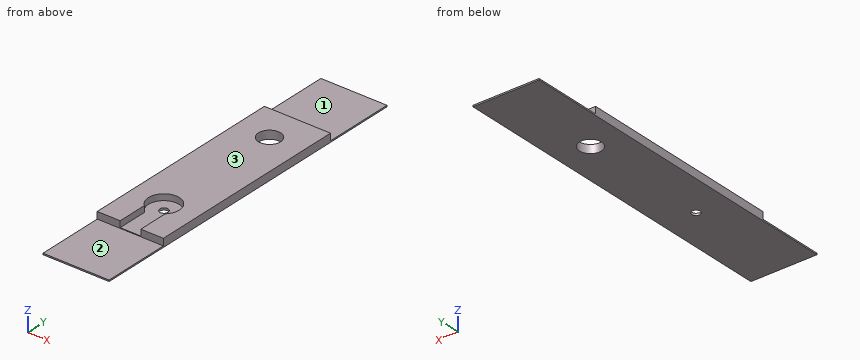
```python
from build123d import *

# Parameters (mm, degrees)
SKETCH_W        = 48
SKETCH_H        = 250.999997
SKETCH_R        = 8.05
SKETCH_R_2      = 3.05
PAD_DEPTH       = 6
POCKET_DEPTH    = 4.5
SKETCH002_W     = 48.1
SKETCH002_H     = 48.999997
POCKET001_DEPTH = 5.001
SKETCH003_W     = 48.1
SKETCH003_H     = 52
POCKET002_DEPTH = 5.001


with BuildPart() as part:
    # Sketch → Pad (new body)
    with BuildSketch(Plane.XY):
        with Locations((-24, 125.499994)):
            Rectangle(SKETCH_W, SKETCH_H)
        with Locations((-24, 174.761047)):
            Circle(SKETCH_R, mode=Mode.SUBTRACT)
        with Locations((-24, 79.409981)):
            Circle(SKETCH_R_2, mode=Mode.SUBTRACT)
    extrude(amount=-PAD_DEPTH)

    # Sketch001 → Pocket (cut)
    with BuildSketch(Plane.XY):
        with BuildLine():
            Line((-31.346662, 47.787562), (-16.346662, 47.787562))
            Line((-16.346662, 47.787562), (-16.346662, 71.017092))
            ThreePointArc((-16.346662, 71.017092), (-24.104532, 90.522743), (-31.346662, 70.819786))
            Line((-31.346662, 70.819786), (-31.346662, 47.787562))
        make_face()
    extrude(amount=-POCKET_DEPTH, mode=Mode.SUBTRACT)

    # Sketch002 → Pocket001 (cut, through all)
    with BuildSketch(Plane.XY.offset(-5)):
        with Locations((-23.95, 24.499994)):
            Rectangle(SKETCH002_W, SKETCH002_H)
    extrude(amount=POCKET001_DEPTH, mode=Mode.SUBTRACT)

    # Sketch003 → Pocket002 (cut, through all)
    with BuildSketch(Plane.XY.offset(-5)):
        with Locations((-23.95, 226)):
            Rectangle(SKETCH003_W, SKETCH003_H)
    extrude(amount=POCKET002_DEPTH, mode=Mode.SUBTRACT)


solid = part.part
```
Geometry check sheet. Reference: the model listing, model coordinates, mm. Face numbers are marked on the shaded views. A direction names the side the tool comes from. Coordinates: 2 decimals unless noted, no trailing zeros. Write each loop counter-clockwise with the first axis right and the second up, starting at its lowest first coordinate (ties: lowest second). Pieces come first, ordered by that corner, then holes. Notation, with made-up numbers: M 87,14 L 128,14 A26 ccw 128,46 Z; hole C -25.5,-15 d2. An arc over 180 degrees is marked long. One line per item, written item: value. Start each with the question number.
(1) Depth check by flat-ended pin: pin 1 (10 mm diameter, centred on x = -24, y = 79.41, fed in from +Z); pin 2 (2 mm diameter, centred on x = -30, z = -1, fed in from +Y); pin 3 (24 mm diameter, centred on x = -12, y = 36.5, fed in from +Z); pin 4 (1.5 mm diameter, centred on y = 48, z = -3, fed in from -X). Enter the tip coordinate at first touch or a pass-through.
(2) Sectioned sample at A-A, the plane x = -24. Enter the section's corners in (y, z).
(3) Scan lines: line 1 along Y through (x, z) = (-24, -5.3); line 2 along Y through (x, z) = (-24, -2.3); line 3 along X through (y, z) = (51, -3.2). Record each from-to range of solid material in increasing order. Write a range as [from, to].
(4) Sectioned sample at B-B, the plane z = -1.2. Enter the section's corners in (x, y), and give its area (3 significant figures).
(5) Sectioned sample at D-D, the plane y = 204.5. Enter the section's corners in (x, z).
(6) Sectioned sample at C-C, the plane x = -39. Enter the section's corners in (y, z), and give its area (3 significant figures).
(7) Tool access check on the marked faces 1, 2 and 3. Record the directions out of +Z, -Z, +X, -X, +Y, -Y that give a thin tool (end or side, any length) a straight path to the whole face; none if there is none.
Filled sheet:
1. pin 1: z = -4.5
1. pin 2: y = 200
1. pin 3: z = -5
1. pin 4: through
2. outline: M 0,-6 L 76.36,-6 L 76.36,-4.5 L 49,-4.5 L 49,-5 L 0,-5 Z; M 82.46,-6 L 166.71,-6 L 166.71,0 L 90.52,0 L 90.52,-4.5 L 82.46,-4.5 Z; M 182.81,-6 L 251,-6 L 251,-5 L 200,-5 L 200,0 L 182.81,0 Z
3. line 1: [0, 76.36], [82.46, 166.71], [182.81, 251]
3. line 2: [90.52, 166.71], [182.81, 200]
3. line 3: [-48, -31.35], [-16.35, 0]
4. outline: M -48,49 L -31.35,49 L -31.35,70.82 A11.24 cw long -16.35,71.02 L -16.35,49 L 0,49 L 0,200 L -48,200 Z; hole C -24,174.76 d16.1
4. area: 6,350 mm²
5. outline: M -48,-6 L 0,-6 L 0,-5 L -48,-5 Z
6. outline: M 0,-6 L 251,-6 L 251,-5 L 200,-5 L 200,0 L 49,0 L 49,-5 L 0,-5 Z
6. area: 1,010 mm²
7. face 1: +Z, +X, -X, +Y
7. face 2: +Z, +X, -X, -Y
7. face 3: +Z, +X, -X, +Y, -Y
